from build123d import *

# Parameters (mm, degrees)
EXTRUDE_1_DEPTH     = 20
SKETCH_2_R          = 1.5
CUT_EXTRUDE_1_DEPTH = 47.519485165
SKETCH_5_W          = 1.5
SKETCH_5_H          = 4.502682252
EXTRUDE_2_DEPTH     = 10
SKETCH_6_R          = 1.5
CUT_EXTRUDE_2_DEPTH = 54.43647957
SKETCH_7_R          = 2
CUT_EXTRUDE_3_DEPTH = 53.126408809
SKETCH_8_R          = 8
CUT_EXTRUDE_4_DEPTH = 10
SKETCH_9_R          = 1.5
CUT_EXTRUDE_5_DEPTH = 54.307080663


with BuildPart() as part:
    # 스케치1 → 보스-돌출1 (new body)
    with BuildSketch(Plane(origin=(0, 0, 0), x_dir=(0, 0, -1), z_dir=(1, 0, 0))):
        with BuildLine():
            ThreePointArc((-12.25, 6.977642868), (-7.631746424, -1.399585383), (-15, -7.5))
            Line((-15, -7.5), (15, -7.5))
            ThreePointArc((15, -7.5), (7.631746424, -1.399585383), (12.25, 6.977642868))
            Line((12.25, 6.977642868), (-12.25, 6.977642868))
        make_face()
        with BuildLine():
            Line((-17.75, 5.332682252), (-17.75, 6.977642868))
            ThreePointArc((-17.75, 6.977642868), (-22.368253576, -1.399585383), (-15, -7.5))
            ThreePointArc((-15, -7.5), (-7.631746424, -1.399585383), (-12.25, 6.977642868))
            Line((-12.25, 6.977642868), (-12.25, 5.332682252))
            ThreePointArc((-12.25, 5.332682252), (-15, -6), (-17.75, 5.332682252))
        make_face()
        with BuildLine():
            ThreePointArc((-13.75, 5.868347297), (-12.982146125, 5.650510219), (-12.25, 5.332682252))
            Line((-12.25, 5.332682252), (-12.25, 6.977642868))
            ThreePointArc((-12.25, 6.977642868), (-12.989137608, 7.225401888), (-13.75, 7.395099729))
            Line((-13.75, 7.395099729), (-13.75, 5.868347297))
        make_face()
        with BuildLine():
            ThreePointArc((-16.25, 7.395099729), (-17.010862392, 7.225401888), (-17.75, 6.977642868))
            Line((-17.75, 6.977642868), (-17.75, 5.332682252))
            ThreePointArc((-17.75, 5.332682252), (-17.017853875, 5.650510219), (-16.25, 5.868347297))
            Line((-16.25, 5.868347297), (-16.25, 7.395099729))
        make_face()
        with BuildLine():
            Line((-16.25, 12), (-17.75, 12))
            Line((-17.75, 12), (-17.75, 6.977642868))
            ThreePointArc((-17.75, 6.977642868), (-17.010862392, 7.225401888), (-16.25, 7.395099729))
            Line((-16.25, 7.395099729), (-16.25, 10.5))
            Line((-16.25, 10.5), (-16.25, 12))
        make_face()
        with BuildLine():
            ThreePointArc((-13.75, 7.395099729), (-12.989137608, 7.225401888), (-12.25, 6.977642868))
            Line((-12.25, 6.977642868), (-12.25, 12))
            Line((-12.25, 12), (-13.75, 12))
            Line((-13.75, 12), (-13.75, 10.5))
            Line((-13.75, 10.5), (-13.75, 7.395099729))
        make_face()
        with BuildLine():
            ThreePointArc((12.25, 6.977642868), (7.631746424, -1.399585383), (15, -7.5))
            ThreePointArc((15, -7.5), (22.368253576, -1.399585383), (17.75, 6.977642868))
            Line((17.75, 6.977642868), (17.75, 5.332682252))
            ThreePointArc((17.75, 5.332682252), (15, -6), (12.25, 5.332682252))
            Line((12.25, 5.332682252), (12.25, 6.977642868))
        make_face()
        with BuildLine():
            Line((17.75, 5.332682252), (17.75, 6.977642868))
            ThreePointArc((17.75, 6.977642868), (17.010862392, 7.225401888), (16.25, 7.395099729))
            Line((16.25, 7.395099729), (16.25, 5.868347297))
            ThreePointArc((16.25, 5.868347297), (17.017853875, 5.650510219), (17.75, 5.332682252))
        make_face()
        with BuildLine():
            ThreePointArc((16.25, 7.395099729), (17.010862392, 7.225401888), (17.75, 6.977642868))
            Line((17.75, 6.977642868), (17.75, 12))
            Line((17.75, 12), (16.25, 12))
            Line((16.25, 12), (16.25, 10.5))
            Line((16.25, 10.5), (16.25, 7.395099729))
        make_face()
        with BuildLine():
            Line((12.25, 12), (12.25, 6.977642868))
            ThreePointArc((12.25, 6.977642868), (12.989137608, 7.225401888), (13.75, 7.395099729))
            Line((13.75, 7.395099729), (13.75, 10.5))
            Line((13.75, 10.5), (13.75, 12))
            Line((13.75, 12), (12.25, 12))
        make_face()
        with BuildLine():
            ThreePointArc((13.75, 7.395099729), (12.989137608, 7.225401888), (12.25, 6.977642868))
            Line((12.25, 6.977642868), (12.25, 5.332682252))
            ThreePointArc((12.25, 5.332682252), (12.982146125, 5.650510219), (13.75, 5.868347297))
            Line((13.75, 5.868347297), (13.75, 7.395099729))
        make_face()
    extrude(amount=EXTRUDE_1_DEPTH)

    # 스케치2 → 컷-돌출1 (cut, through all)
    with BuildSketch(Plane.XY.offset(17.75)):
        with Locations((3.5, 9.488821434)):
            Circle(SKETCH_2_R)
        with Locations((10, 9.488821434)):
            Circle(SKETCH_2_R)
        with Locations(Location((16.5, 9.488821434, 0), (0, 0, 90))):
            Circle(SKETCH_2_R)
    extrude(amount=-CUT_EXTRUDE_1_DEPTH, mode=Mode.SUBTRACT)

    # 스케치5 → 보스-돌출2 (add, symmetric)
    with BuildSketch(Plane.XY):
        with BuildLine():
            ThreePointArc((32.5, -15), (30.303300859, -9.696699141), (25, -7.5))
            ThreePointArc((25, -7.5), (17.631746424, -13.600414617), (22.25, -21.977642868))
            Line((22.25, -21.977642868), (22.25, -20.332682252))
            ThreePointArc((22.25, -20.332682252), (21.877501001, -9.876524617), (31, -15))
            ThreePointArc((31, -15), (30.123475383, -18.122498999), (27.75, -20.332682252))
            Line((27.75, -20.332682252), (27.75, -21.977642868))
            ThreePointArc((27.75, -21.977642868), (31.199798384, -19.220485754), (32.5, -15))
        make_face()
        with BuildLine():
            Line((22.25, -20.332682252), (22.25, -21.977642868))
            ThreePointArc((22.25, -21.977642868), (22.989137608, -22.225401888), (23.75, -22.395099729))
            Line((23.75, -22.395099729), (23.75, -20.868347297))
            ThreePointArc((23.75, -20.868347297), (22.982146125, -20.650510219), (22.25, -20.332682252))
        make_face()
        with BuildLine():
            ThreePointArc((26.25, -22.395099729), (27.010862392, -22.225401888), (27.75, -21.977642868))
            Line((27.75, -21.977642868), (27.75, -20.332682252))
            ThreePointArc((27.75, -20.332682252), (27.017853875, -20.650510219), (26.25, -20.868347297))
            Line((26.25, -20.868347297), (26.25, -22.395099729))
        make_face()
        with BuildLine():
            Line((27.75, -27.002682252), (27.75, -21.977642868))
            ThreePointArc((27.75, -21.977642868), (27.010862392, -22.225401888), (26.25, -22.395099729))
            Line((26.25, -22.395099729), (26.25, -27.002682252))
            Line((26.25, -27.002682252), (27.75, -27.002682252))
        make_face()
        with BuildLine():
            ThreePointArc((23.75, -22.395099729), (22.989137608, -22.225401888), (22.25, -21.977642868))
            Line((22.25, -21.977642868), (22.25, -22.5))
            Line((22.25, -22.5), (23.75, -22.5))
            Line((23.75, -22.5), (23.75, -22.395099729))
        make_face()
        with Locations((23, -24.751341126)):
            Rectangle(SKETCH_5_W, SKETCH_5_H)
        with BuildLine():
            ThreePointArc((22.25, -21.977642868), (17.631746424, -13.600414617), (25, -7.5))
            Line((25, -7.5), (20, -7.5))
            Line((20, -7.5), (0, -7.5))
            Line((0, -7.5), (-5, -7.5))
            ThreePointArc((-5, -7.5), (0.303300859, -9.696699141), (2.5, -15))
            ThreePointArc((2.5, -15), (1.199798384, -19.220485754), (-2.25, -21.977642868))
            Line((-2.25, -21.977642868), (-2.25, -22.5))
            Line((-2.25, -22.5), (22.25, -22.5))
            Line((22.25, -22.5), (22.25, -21.977642868))
        make_face()
        with BuildLine():
            ThreePointArc((2.5, -15), (0.303300859, -9.696699141), (-5, -7.5))
            ThreePointArc((-5, -7.5), (-12.368253576, -13.600414617), (-7.75, -21.977642868))
            Line((-7.75, -21.977642868), (-7.75, -20.332682252))
            ThreePointArc((-7.75, -20.332682252), (-8.122498999, -9.876524617), (1, -15))
            ThreePointArc((1, -15), (0.123475383, -18.122498999), (-2.25, -20.332682252))
            Line((-2.25, -20.332682252), (-2.25, -21.977642868))
            ThreePointArc((-2.25, -21.977642868), (1.199798384, -19.220485754), (2.5, -15))
        make_face()
        with BuildLine():
            Line((-7.75, -20.332682252), (-7.75, -21.977642868))
            ThreePointArc((-7.75, -21.977642868), (-7.010862392, -22.225401888), (-6.25, -22.395099729))
            Line((-6.25, -22.395099729), (-6.25, -20.868347297))
            ThreePointArc((-6.25, -20.868347297), (-7.017853875, -20.650510219), (-7.75, -20.332682252))
        make_face()
        with BuildLine():
            ThreePointArc((-6.25, -22.395099729), (-7.010862392, -22.225401888), (-7.75, -21.977642868))
            Line((-7.75, -21.977642868), (-7.75, -27.002682252))
            Line((-7.75, -27.002682252), (-6.25, -27.002682252))
            Line((-6.25, -27.002682252), (-6.25, -22.395099729))
        make_face()
        with BuildLine():
            Line((-3.75, -22.5), (-2.25, -22.5))
            Line((-2.25, -22.5), (-2.25, -21.977642868))
            ThreePointArc((-2.25, -21.977642868), (-2.989137608, -22.225401888), (-3.75, -22.395099729))
            Line((-3.75, -22.395099729), (-3.75, -22.5))
        make_face()
        with Locations((-3, -24.751341126)):
            Rectangle(SKETCH_5_W, SKETCH_5_H)
        with BuildLine():
            ThreePointArc((-3.75, -22.395099729), (-2.989137608, -22.225401888), (-2.25, -21.977642868))
            Line((-2.25, -21.977642868), (-2.25, -20.332682252))
            ThreePointArc((-2.25, -20.332682252), (-2.982146125, -20.650510219), (-3.75, -20.868347297))
            Line((-3.75, -20.868347297), (-3.75, -22.395099729))
        make_face()
    extrude(amount=EXTRUDE_2_DEPTH, both=True)

    # 스케치6 → 컷-돌출2 (cut, through all)
    with BuildSketch(Plane(origin=(27.75, 0, 0), x_dir=(0, 0, -1), z_dir=(1, 0, 0))):
        with Locations((-6.5, -24.49016256)):
            Circle(SKETCH_6_R)
        with Locations((0, -24.49016256)):
            Circle(SKETCH_6_R)
        with Locations((6.5, -24.49016256)):
            Circle(SKETCH_6_R)
    extrude(amount=-CUT_EXTRUDE_2_DEPTH, mode=Mode.SUBTRACT)

    # 스케치7 → 컷-돌출3 (cut, through all)
    with BuildSketch(Plane(origin=(0, 6.977642868, 0), x_dir=(1, 0, 0), z_dir=(0, 1, 0))):
        with Locations(Location((10, 0, 0), (0, 0, 270))):
            Circle(SKETCH_7_R)
    extrude(amount=-CUT_EXTRUDE_3_DEPTH, mode=Mode.SUBTRACT)

    # 스케치8 → 컷-돌출4 (cut)
    with BuildSketch(Plane.XZ.offset(22.5)):
        with Locations(Location((10, 0, 0), (0, 0, 270))):
            Circle(SKETCH_8_R)
    extrude(amount=-CUT_EXTRUDE_4_DEPTH, mode=Mode.SUBTRACT)

    # 스케치9 → 컷-돌출5 (cut, through all)
    with BuildSketch(Plane.XY.offset(10)):
        with Locations((17.5, -18.8)):
            Circle(SKETCH_9_R)
        with Locations((2.5, -18.8)):
            Circle(SKETCH_9_R)
    extrude(amount=-CUT_EXTRUDE_5_DEPTH, mode=Mode.SUBTRACT)


solid = part.part
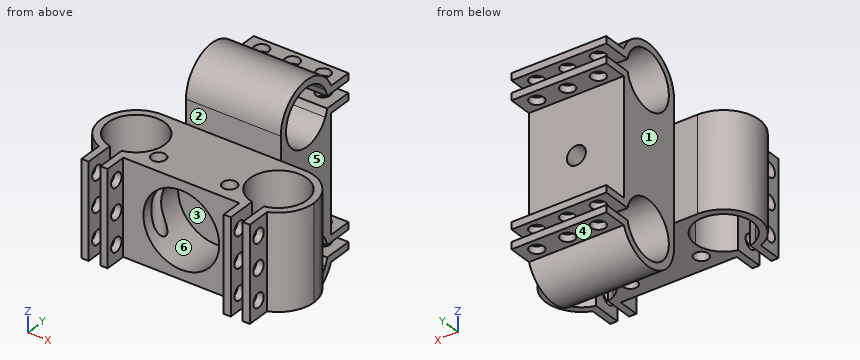
Here's how the part is built. I have some questions about the finished solid (model axes, mm). Face numbers are marked on the shaded views. A direction names the side the tool comes from. Coordinates: 2 decimals unless noted, no trailing zeros. Write each loop counter-clockwise with the first axis right and the second up, starting at its lowest first coordinate (ties: lowest second). Pieces come first, ordered by that corner, then holes.
Item 1: If I drill on line 1 (X direction, y = -17, z = 6.5); line 2 (Z direction, x = 17, y = 1); line 3 (Y direction, x = 23.1, z = 0), over which ranges is the centre line in solid material (lowest first)?
Item 2: I want a section at C-C on z = -6.5. Count the separate pieces of the cut face and the enclosed holes in it, and give its area (3 significant figures).
Item 3: I want a section at D-D on y = -5. Write out the boundary of the cut face in (x, z).
Item 4: On a 3-axis mill with a long thin cutter (end or side, diameter ignored), from which of +Z, -Z, +X, -X, +Y, -Y can I reach the whole of each face in a straight line? I mean the marked faces 1, 2 and 3. Say none if no direction works.
Item 5: If we mould it in two halves opening along X, with no side actions, what happens to the marked faces 4, 5 and 6? For each: +X half, -X half, draft (parallel to the pull), parting line (faces both ways), or undercut.
Item 6: I want a section at A-A on y = 0. Write out the boundary of the cut face in (x, z).
Item 7: Will these pins go through, and if not, where does the flat tip stop? pin 1 (1.8 mm diameter, centred on x = 8, y = 8, fed in from +Z); pin 2 (1.5 mm diameter, centred on x = 22.5, z = -3, fed in from +Y); pin 3 (4 mm diameter, centred on x = 10, y = 9.49, fed in from -Z); pin 4 (2.5 mm diameter, centred on y = -24.49, z = 0, fed in from +X).
Item 8: I want a section at B-B on y = -18.8. Write out the boundary of the cut face in (x, z).
Findings below:
1. line 1: x = -12.23 to -10.66, 0.66 to 5.34, 14.66 to 19.34, 30.66 to 32.23
1. line 2: z = -22.43 to -20.92, -9.08 to 9.08, 20.92 to 22.43
1. line 3: y = -27 to -25.99, -22.99 to -20.69, -9.31 to -7.5
2. separate pieces: 5
2. enclosed holes: 2
2. area: 585 mm2
3. outline: (0, -20.59) - (20, -20.59) - (20, -18.32) - (0, -18.32) - close; (0, -11.68) - (20, -11.68) - (20, 11.68) - (0, 11.68) - close; (0, 18.32) - (20, 18.32) - (20, 20.59) - (0, 20.59) - close; hole circle Ø4 at (10, 0)
4. face 1: +Z, -Z, -X, +Y
4. face 2: +Z, +X, -X, -Y
4. face 3: -Y
5. face 4: draft
5. face 5: +X half
5. face 6: undercut
6. outline: (0, -22.5) - (20, -22.5) - (20, -21) - (0, -21) - close; (0, -9) - (20, -9) - (20, 9) - (0, 9) - close; (0, 21) - (20, 21) - (20, 22.5) - (0, 22.5) - close; hole circle Ø4 at (10, 0)
7. pin 1: stops at z = 17.75
7. pin 2: stops at y = -7.5
7. pin 3: stops at z = -17.75
7. pin 4: passes through
8. outline: (-11.47, -10) - (-9.64, -10) - (-9.64, 10) - (-11.47, 10) - close; (-0.36, -10) - (1, -10) - (1, 10) - (-0.36, 10) - close; (4, -10) - (16, -10) - (16, -5.29) arc R8 cw to (4, -5.29) - close; (4, 5.29) arc R8 cw to (16, 5.29) - (16, 10) - (4, 10) - close; (19, -10) - (20.36, -10) - (20.36, 10) - (19, 10) - close; (29.64, -10) - (31.47, -10) - (31.47, 10) - (29.64, 10) - close
